from build123d import *

# Parameters (mm, degrees)
F0_R     = 6.1
F1_DEPTH = 25
F2_R     = 2.3
F3_DEPTH = 25
F4_DEPTH = 2
F5_D     = 3.3


with BuildPart() as f1:
    # F0 (on Top) → F1 (new body)
    with BuildSketch(Plane.XY):
        with BuildLine():
            ThreePointArc((2.1, -6.7823299831), (5.7148928249, -4.2130748866), (7.1, 0))
            ThreePointArc((7.1, 0), (-5.7148928249, 4.2130748866), (2.1, -6.7823299831))
        make_face()
        Circle(F0_R, mode=Mode.SUBTRACT)
        with BuildLine():
            Line((7.1, -17), (7.1, 0))
            ThreePointArc((7.1, 0), (5.7148928249, -4.2130748866), (2.1, -6.7823299831))
            Line((2.1, -6.7823299831), (2.1, -17))
            Line((2.1, -17), (7.1, -17))
        make_face()
    extrude(amount=F1_DEPTH)

    # F2 (on face) → F3 (cut)
    with BuildSketch(Plane(origin=(2.1, 0, 0), x_dir=(0, -1, 0), z_dir=(-1, 0, 0))):
        with BuildLine():
            ThreePointArc((6.7823299831, 16.9879498806), (9.0729868094, 17.0039599884), (10.2137183353, 18.9904384315))
            ThreePointArc((10.2137183353, 18.9904384315), (9.0729868094, 20.9769168746), (6.7823299831, 20.9929269824))
            Line((6.7823299831, 20.9929269824), (6.7823299831, 16.9879498806))
        make_face()
        with Locations((7.9137183353, 18.9904384315)):
            Circle(F2_R)
        with Locations((7.9137183353, 7.0155123249)):
            Circle(F2_R)
    extrude(amount=F3_DEPTH, mode=Mode.SUBTRACT)

    # F2 (on face) → F4 (cut)
    with BuildSketch(Plane(origin=(2.1, 0, 0), x_dir=(0, -1, 0), z_dir=(-1, 0, 0))):
        with Locations((7.9137183353, 18.9904384315)):
            Circle(F2_R)
        with Locations((7.9137183353, 7.0155123249)):
            Circle(F2_R)
    extrude(amount=-F4_DEPTH, mode=Mode.SUBTRACT)

    # F5 (through all)
    with Locations(Plane(origin=(2.1, 0, 0), x_dir=(0, -1, 0), z_dir=(-1, 0, 0))):
        with Locations((7.9137183353, 7.0155123249), (7.9137183353, 18.9904384315)):
            Hole(F5_D / 2)


solid = f1.part
The model under review builds one solid part; all positions refer to its coordinate system, in mm. A direction names the side the tool comes from. Round coordinates to 2 decimals unless told otherwise and drop trailing zeros. Order: outer loops, then holes, each group sorted by start corner. A loop starts at its lowest first (then second) coordinate and runs counter-clockwise, first axis right, second up. Notation, with made-up numbers: (12, 73.5) - (62, 73.5) arc R17 cw to (62, 80.5) - close; hole circle Ø7 at (-2.5, 77.5). An arc over 180 degrees is marked (long way). Use one line per item in the form item = value.
Q1. Add section A-A on x = 3. Give the boundary of the cut face in (y, z).
Response values:
outline = (-17, 0) - (-5.31, 0) - (-5.31, 25) - (-17, 25) - close; (5.31, 0) - (6.44, 0) - (6.44, 25) - (5.31, 25) - close; hole circle Ø4.6 at (-7.91, 7.02); hole circle Ø4.6 at (-7.91, 18.99)
Q2. Add section D-D on y = -4.75. Give the boundary of the cut face in (x, z), then the cut area to 3 significant figures.
Response values:
outline = (-5.28, 0) - (-3.83, 0) - (-3.83, 25) - (-5.28, 25) - close; (3.83, 0) - (7.1, 0) - (7.1, 25) - (3.83, 25) - close
area = 118 mm^2
Q3. Tool access review of faces 4 (the flat face through (4.1, -9.4, 6)), 5 (the cylindrical face through (5.621, -9.13, 20.106)): name each direction out of +Z, -Z, +X, -X, +Y, -Y from which nothing blocks a thin tool from reaching the whole face with its end or side.
Response values:
face_4 = -X
face_5 = +X, -X
Q4. To check wall thickness, follow line 1 (Y direction, x = 3, z = 18); line 2 (Y direction, x = 3.25, z = 9); line 3 (Y direction, x = 0.25, z = 11.5). State the ranges of each line that lie inside material, in increasing order.
Response values:
line_1 = -17 to -9.99, -5.84 to -5.31, 5.31 to 6.44
line_2 = -17 to -9.08, -6.75 to -5.16, 5.16 to 6.31
line_3 = -7.1 to -6.09, 6.09 to 7.1
Q5. Add section B-B on z = 5.75. Give the boundary of the cut face in (x, y), then the cut area to 3 significant figures.
Response values:
outline = (-3.81, -5.99) - (-1.14, -5.99) arc R6.1 cw (long way) to (1.14, -5.99) - (4.1, -5.99) - (4.1, -6.85) - (7.1, -6.85) - (7.1, 0) arc R7.1 ccw (long way) to start; (2.1, -17) - (7.1, -17) - (7.1, -8.97) - (4.1, -8.97) - (4.1, -9.83) - (2.1, -9.83) - close
area = 82.7 mm^2
Q6. Mouldability with a two-part tool opening along X and no side actions: class faces 1 (the cylindrical face through (3.279, 5.144, 12.325)), 2 (the flat face through (7.1, -9, 12)), 3 (the cylindrical face through (5.621, -9.562, 7.088)) as pulls with the +X half, pulls with the -X half, needs draft (parallel to the pull), parting line crosses it, or undercut.
Response values:
face_1 = undercut
face_2 = pulls with the +X half
face_3 = needs draft
Q7. Add section C-C on x = 0. Give the boundary of the cut face in (y, z), then the cut area to 3 significant figures.
Response values:
outline = (-7.1, 0) - (-6.1, 0) - (-6.1, 5.6) arc R2.3 cw to (-7.1, 4.86) - close; (-7.1, 9.17) arc R2.3 cw to (-6.1, 8.43) - (-6.1, 17.58) arc R2.3 cw to (-7.1, 16.84) - close; (-7.1, 21.14) arc R2.3 cw to (-6.1, 20.4) - (-6.1, 25) - (-7.1, 25) - close; (6.1, 0) - (7.1, 0) - (7.1, 25) - (6.1, 25) - close
area = 42.6 mm^2
Q8. Clearance check with flat-ended pins moving along their axes: P1, Ø1.4, axis at y = -8, z = 8, coming from the -X side; P2, Ø2, axis at x = -1.5, z = 13, coming from the -Y side; P3, Ø7.5, axis at x = 0, y = 0, coming from the -Z side; P4, Ø8, axis at y = -5, z = 11, coming from the -X side. State where each tip first meets the part, or that it passes through.
Response values:
P1 = 4.1
P2 = -7.08
P3 = through
P4 = -7.03
